Design review of the part shown in the three views and the two pictorial views. Dimensions are in mm from the part's minimum x, y and z. A direction names the side the tool comes from. Coordinates: 2 decimals unless noted, no trailing zeros. Order: outer loops, then holes, each group sorted by start corner. A loop starts at its lowest first (then second) coordinate and runs counter-clockwise, first axis right, second up. Notation, with made-up numbers: (-19.5, -6) -> (2.5, -6) arc R17 cw to (2.5, 26) -> close; hole circle Ø1 at (-16, 42). An arc over 180 degrees is marked (long way). Answer as a JSON object with one key per item and string values. Group by question number.
1) Add section A-A, the plane x = 28.5. Write out the cut boundary in (y, z).
2) Add section D-D, the plane y = 3. Write out the cut boundary in (x, z).
3) Wall thickness on L1, parallel to Z at x = 15, y = 8; L2, parallel to X at y = 5.5, z = 80.5; L3, parallel to X at y = 12, z = 15.5: over which ranges is each line inside the solid? List them lowest first.
4) Machinability: for the marked faces 1 and 2, which of the approach directions +Z, -Z, +X, -X, +Y, -Y give a long, thin tool a straight path to every point of the face, cutting with its end or side? Answer none if there is none.
5) For pin 1 (8 mm diameter, centred on x = 16, z = 19, fed in from -Y); pin 2 (1.5 mm diameter, centred on y = 7.5, z = 29.5, fed in from +X); pin 3 (4 mm diameter, centred on y = 9.5, z = 32.5, fed in from -X), all flat-tipped, find the tip position at first contact; note any pin that passes through.
6) Add section C-C, the plane z = 17. Write out the cut boundary in (x, y), then the cut area to 3 significant figures.
7) Add section B-B, the plane y = 9. Write out the cut boundary in (x, z), then the cut area to 3 significant figures.
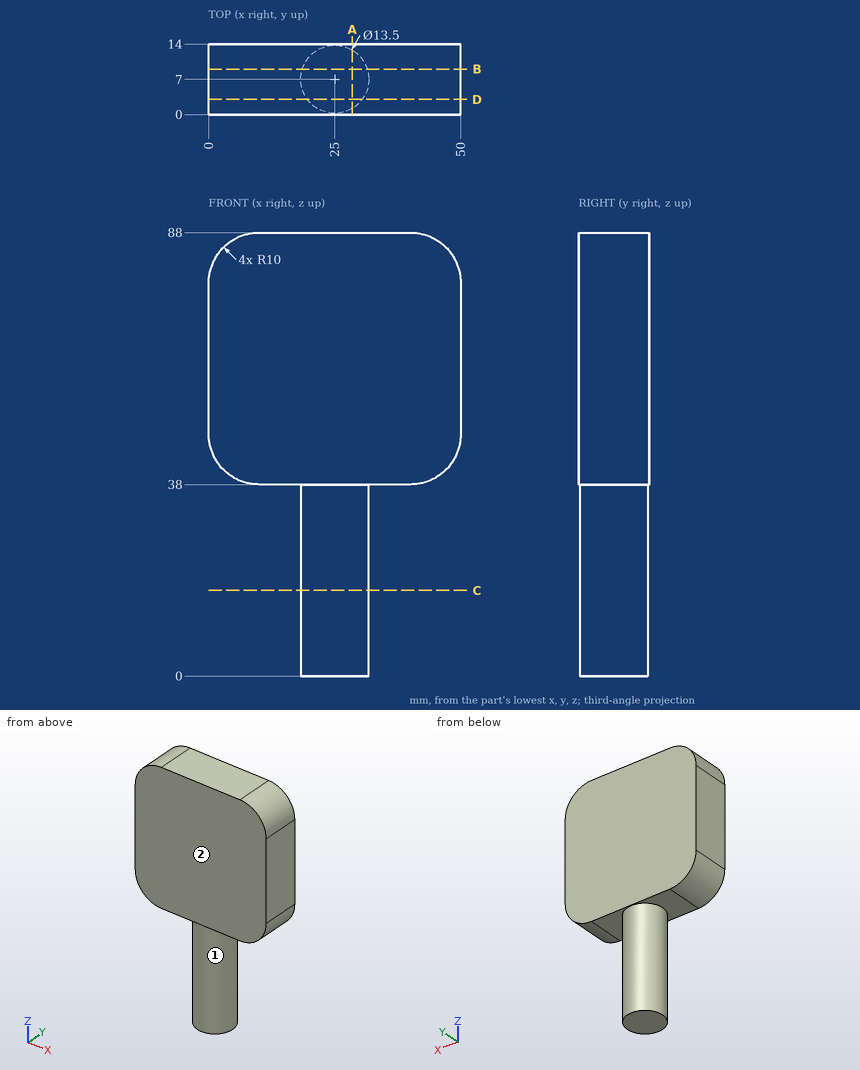
Output values:
{
 "1": {"outline": "(0, 38) -> (1.23, 38) -> (1.23, 0) -> (12.77, 0) -> (12.77, 38) -> (14, 38) -> (14, 88) -> (0, 88) -> close"},
 "2": {"outline": "(0, 48) arc R10 ccw to (10, 38) -> (19.56, 38) -> (19.56, 0) -> (30.44, 0) -> (30.44, 38) -> (40, 38) arc R10 ccw to (50, 48) -> (50, 78) arc R10 ccw to (40, 88) -> (10, 88) arc R10 ccw to (0, 78) -> close"},
 "3": {"L1": "z = 38 to 88", "L2": "x = 0.32 to 49.68", "L3": "x = 20.47 to 29.53"},
 "4": {"face 1": "-Z", "face 2": "+Z, -Z, +X, -X, -Y"},
 "5": {"pin 1": "stops at y = 2.47", "pin 2": "stops at x = 31.75", "pin 3": "stops at x = 18.27"},
 "6": {"outline": "circle Ø13.5 at (25, 7)", "area": "143 mm²"},
 "7": {"outline": "(0, 48) arc R10 ccw to (10, 38) -> (18.55, 38) -> (18.55, 0) -> (31.45, 0) -> (31.45, 38) -> (40, 38) arc R10 ccw to (50, 48) -> (50, 78) arc R10 ccw to (40, 88) -> (10, 88) arc R10 ccw to (0, 78) -> close", "area": "2,900 mm²"}
}
